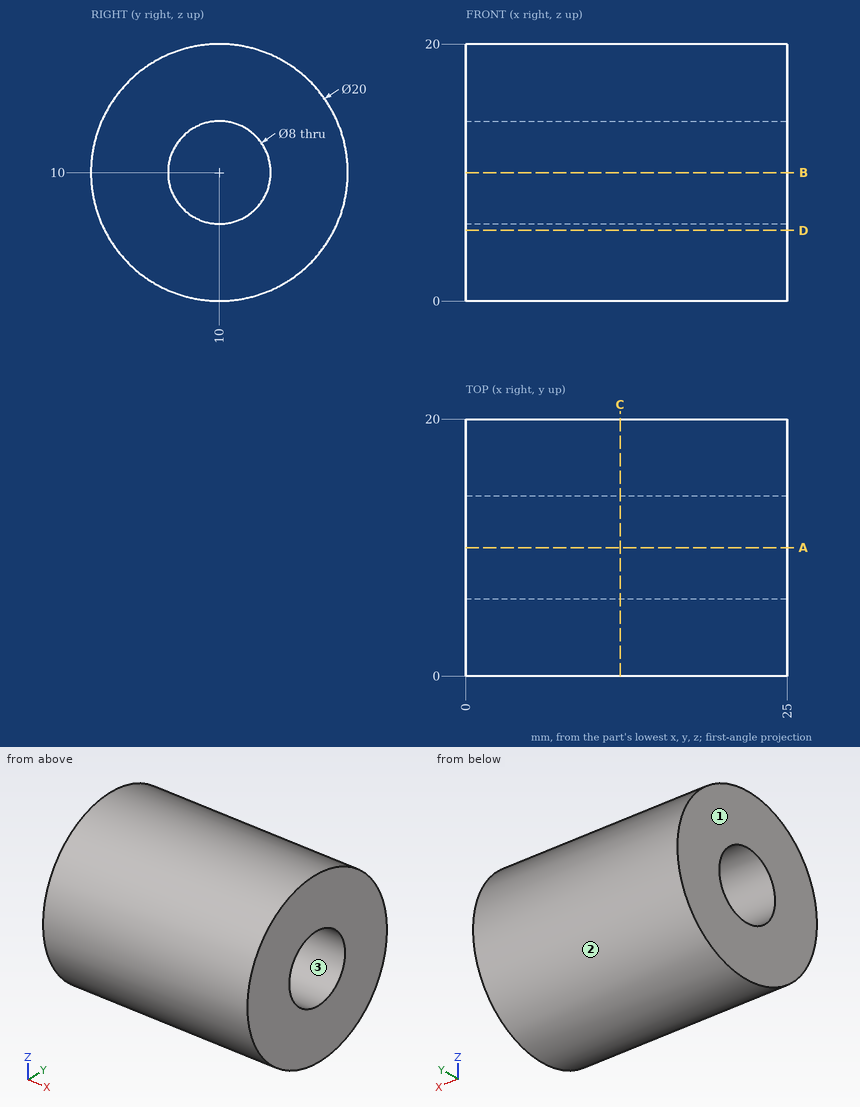
Check sheet for the drawn part. Datum: minimum x, y, z corner. Units: mm. Coordinates: 2 decimals unless noted, no trailing zeros. Order: outer loops, then holes, each group sorted by start corner. A loop starts at its lowest first (then second) coordinate and runs counter-clockwise, first axis right, second up. Notation, with made-up numbers: (12, 32) -> (17, 32) arc R16 ccw to (17, 58) -> close; hole circle Ø5 at (17.5, -29). An arc over 180 degrees is marked (long way). Use a Markdown table: item, result. Add a question column.
1. Material ranges on L1, parallel to Z at x = 13.75, y = 10; L2, parallel to Y at x = 14.5, z = 13.5; L3, parallel to Y at x = 8.75, z = 12.75, recorded low to high.
2. Mould release check, pull along Y, two halves, no side actions. Record for the marked faces 1, 2 and 3: pulls with the +Y half, pulls with the -Y half, needs draft (parallel to the pull), parting line crosses it, or undercut.
3. Cross-section at C-C (x = 12). Enter the section's corners in (y, z), and give its area (3 significant figures).
4. Go/stop test with flat-tipped pins: pin 1 Ø8 at (x, y) = (18.5, 18) entering from +Z; pin 2 Ø5 at (x, y) = (11, 5) entering from +Z; pin 3 Ø5 at (x, y) = (22, 6) entering from +Z. Record where each tip stops, or that it passes through.
5. Cross-section at D-D (z = 5.5). Enter the section's corners in (x, y), and give its area (3 significant figures).
6. Cross-section at A-A (y = 10). Enter the section's corners in (x, z).
Filled sheet:
| question | item | result |
|---|---|---|
| 1 | L1 | 0 to 6, 14 to 20 |
| 1 | L2 | 0.63 to 8.06, 11.94 to 19.37 |
| 1 | L3 | 0.39 to 7.1, 12.9 to 19.61 |
| 2 | face 1 | needs draft |
| 2 | face 2 | parting line crosses it |
| 2 | face 3 | undercut |
| 3 | outline | circle Ø20 at (10, 10); hole circle Ø8 at (10, 10) |
| 3 | area | 264 mm2 |
| 4 | pin 1 | z = 19.17 |
| 4 | pin 2 | z = 19.68 |
| 4 | pin 3 | z = 19.89 |
| 5 | outline | (0, 1.07) -> (25, 1.07) -> (25, 18.93) -> (0, 18.93) -> close |
| 5 | area | 447 mm2 |
| 6 | outline | (0, 0) -> (25, 0) -> (25, 6) -> (0, 6) -> close; (0, 14) -> (25, 14) -> (25, 20) -> (0, 20) -> close |
